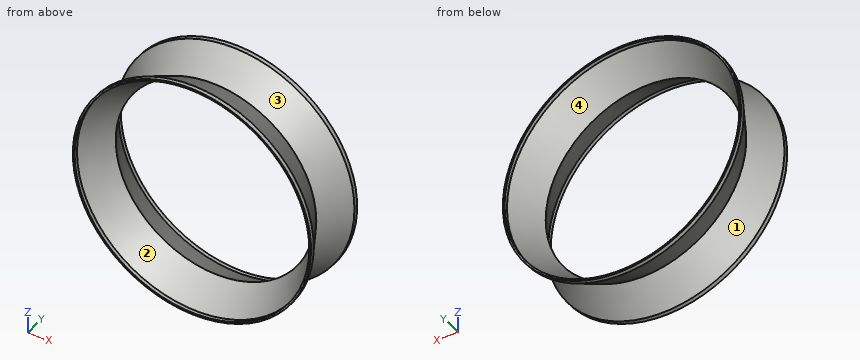
```python
from build123d import *

# Parameters (mm, degrees)
SKETCH_1_R      = 34.670752002
EXTRUDE_1_DEPTH = 1.2
SKETCH_3_R      = 34.670752002
SKETCH_2_R      = 29.48320138


# Read off the part's stored shape, not the designer's step: 쉘1
with BuildPart() as part:
    # 스케치1 → 보스-돌출1 (new body)
    with BuildSketch(Plane(origin=(0, 0, 0), x_dir=(1, 0, 0), z_dir=(0, 1, 0))):
        with Locations(Location((0, 0, 0), (0, 0, 270))):
            Circle(SKETCH_1_R)
    extrude_1 = extrude(amount=EXTRUDE_1_DEPTH)

    # 스케치3 → 로프트1 section 0
    with BuildSketch(Plane(origin=(0, 1.2, 0), x_dir=(1, 0, 0), z_dir=(0, 1, 0))):
        Circle(SKETCH_3_R)
    # 스케치2 → 로프트1 section 1
    with BuildSketch(Plane(origin=(0, 10.2, 0), x_dir=(1, 0, 0), z_dir=(0, 1, 0))):
        Circle(SKETCH_2_R)
    loft_1 = loft()

    # 대칭 복사1: 보스-돌출1, 로프트1 across plane
    add(extrude_1.mirror(Plane.ZX.offset(10.2)))
    add(loft_1.mirror(Plane.ZX.offset(10.2)))

    # 쉘1 outline → 쉘1 (revolve, cut)
    with BuildSketch(Plane.XY):
        Polygon((34.170752002, 0), (34.170752002, 1.066217535), (28.906089901, 10.2), (34.170752002, 19.333782465), (34.170752002, 20.4), (0, 20.4), (0, 0), align=None)
    revolve(axis=Axis((0, 0, 0), (0, 1, 0)), mode=Mode.SUBTRACT)


solid = part.part
```
Geometry check sheet. Reference: the model listing, model coordinates, mm. Face numbers are marked on the shaded views. A direction names the side the tool comes from. Round coordinates to 2 decimals unless told otherwise and drop trailing zeros. Order: outer loops, then holes, each group sorted by start corner. A loop starts at its lowest first (then second) coordinate and runs counter-clockwise, first axis right, second up. Notation, with made-up numbers: (65.5, 6.25) - (96.5, 6.25) arc R11 cw to (96.5, 22.25) - close; hole circle Ø7 at (50.5, 79). An arc over 180 degrees is marked (long way). Use a Markdown table: item, result. Add a question column.
1) Thickness scan on line 1 along X through (y, z) = (20.1, 0); line 2 along Y through (x, z) = (-29.5, -1.5). Record the ranges inside material, lowest first.
2) Gauge pin test, flat ends, axial feed: P1, Ø1, axis at y = 6, z = -16, coming from the -X side; P2, Ø4, axis at x = -17, y = 9.5, coming from the +Z side (3 decimals); P3, Ø8, axis at y = 11.5, z = 26, coming from the +X side. Record the tip position at first contact, or that the pin passes through.
3) Mould release check, pull along Z, two halves, no side actions. Record for the marked faces 1 and 2: released by +Z, released by -Z, zero draft, split by the parting line, or undercut.
4) Set-up check for the marked faces 3 and 4: record each of +Z, -Z, +X, -X, +Y, -Y from which the full face is reachable in a straight line by a thin tool's end or side.
5) Section check B-B (y = 6.75). Record the cut outline in (x, z).
Established:
| question | item | result |
|---|---|---|
| 1 | line 1 | -34.67 to -34.17, 34.17 to 34.67 |
| 1 | line 2 | 9.1 to 10.1, 10.3 to 11.3 |
| 2 | P1 | x = -28.04 |
| 2 | P2 | z = 26.455 |
| 2 | P3 | x = 21.91 |
| 3 | face 1 | split by the parting line |
| 3 | face 2 | undercut |
| 4 | face 3 | none |
| 4 | face 4 | +Y |
| 5 | outline | circle Ø62.94 at (0, 0); hole circle Ø61.79 at (0, 0) |
